```python
from build123d import *

# Parameters (mm, degrees)
SKETCH2_W               = 150
SKETCH2_H               = 80
BOSS_EXTRUDE1_DEPTH     = 3
CUT_EXTRUDE1_DEPTH      = 86.211501571
CUT_EXTRUDE1_DEPTH_BACK = 86.211501571
SKETCH3_R               = 3.25
FILLET2_R               = 8


with BuildPart() as part:
    # Sketch2 → Boss-Extrude1 (new, symmetric)
    with BuildSketch(Plane.XY):
        Rectangle(SKETCH2_W, SKETCH2_H)
    extrude(amount=BOSS_EXTRUDE1_DEPTH, both=True)

    # Sketch3 → Cut-Extrude1 (cut, two sides: drawn at the far end of the back side and taken through both)
    with BuildSketch(Plane.XY.offset(3).offset(-CUT_EXTRUDE1_DEPTH_BACK)):
        with Locations((-60, 28)):
            Circle(SKETCH3_R)
        with Locations((-60, -28)):
            Circle(SKETCH3_R)
        with Locations((60, -28)):
            Circle(SKETCH3_R)
        with Locations((60, 28)):
            Circle(SKETCH3_R)
    extrude(amount=CUT_EXTRUDE1_DEPTH + CUT_EXTRUDE1_DEPTH_BACK, mode=Mode.SUBTRACT)

    # Fillet2
    fillet2_edges = [part.edges().sort_by_distance(p)[0] for p in [
        (75, -40, 0),
        (-75, -40, 0),
        (-75, 40, 0),
        (75, 40, 0),
    ]]
    fillet(fillet2_edges, radius=FILLET2_R)


solid = part.part
```
Could you check a few things on this model? Use its own coordinates, in mm. Coordinates: 2 decimals unless noted, no trailing zeros. Write each loop counter-clockwise with the first axis right and the second up, starting at its lowest first coordinate (ties: lowest second). Pieces come first, ordered by that corner, then holes. Notation, with made-up numbers: M 10.5,38 L 63.5,38 A27 ccw 63.5,58 Z; hole C 25,-25 d2. An arc over 180 degrees is marked long. Answer as CSV lines item,"result". Start each with the question number.
1) I want a section at A-A, the plane x = -60. Please give me the cut outline in (y, z), and give its area (3 significant figures).
2) We'd pull the mould along X, two halves only. Please class faces 1 (the cylindrical face through (72.594, -37.719, 0.042)), 2 (the flat face through (-1, 1, 3)), 3 (the cylindrical face through (-62.579, 26.022, -0.042)): +X half, -X half, draft (parallel to the pull), parting line (faces both ways), or undercut.
3) Please list where these lines run through material, in increasing order: line 1 (Y direction, x = -60, z = 0.85); line 2 (X direction, y = -28, z = 1.1); line 3 (X direction, y = 34, z = -2.2). Write a range as from..to.
4) I want a section at C-C, the plane z = 0.95. Please give me the cut outline in (x, y).
5) For P1, Ø10.5, axis at x = 60, y = 28, coming from the -Z side, with a flat end and sliding along its axis, tell me the tip position at first contact or that it passes through.
6) I want a section at B-B, the plane y = -28. Please give me the cut outline in (x, z).
Data:
1,outline,"M -40,-3 L -31.25,-3 L -31.25,3 L -40,3 Z; M -24.75,-3 L 24.75,-3 L 24.75,3 L -24.75,3 Z; M 31.25,-3 L 40,-3 L 40,3 L 31.25,3 Z"
1,area,"402 mm^2"
2,face 1,"+X half"
2,face 2,"draft"
2,face 3,"undercut"
3,line 1,"y = -40..-31.25, -24.75..24.75, 31.25..40"
3,line 2,"x = -75..-63.25, -56.75..56.75, 63.25..75"
3,line 3,"x = -74.75..74.75"
4,outline,"M -75,-32 A8 ccw -67,-40 L 67,-40 A8 ccw 75,-32 L 75,32 A8 ccw 67,40 L -67,40 A8 ccw -75,32 Z; hole C -60,-28 d6.5; hole C -60,28 d6.5; hole C 60,-28 d6.5; hole C 60,28 d6.5"
5,P1,"stops at z = -3"
6,outline,"M -75,-3 L -63.25,-3 L -63.25,3 L -75,3 Z; M -56.75,-3 L 56.75,-3 L 56.75,3 L -56.75,3 Z; M 63.25,-3 L 75,-3 L 75,3 L 63.25,3 Z"
